Geometry check sheet. Reference: the model listing, model coordinates, mm. A direction names the side the tool comes from. Round coordinates to 2 decimals unless told otherwise and drop trailing zeros. Loops run counter-clockwise (first coordinate to the right, second up) from the corner with the lowest first, then second, coordinate; pieces in that order, holes last. Notation, with made-up numbers: M 54.5,34 L 73.5,34 A19 ccw 73.5,65 Z; hole C -1,-21 d11. An arc over 180 degrees is marked long. Answer in a Markdown table with one row per item. Add a question column.
```python
from build123d import *

# Parameters (mm, degrees)
SKETCH1_R                = 9
SKETCH1_R_2              = 7
BOSS_EXTRUDE1_DEPTH      = 25
CUT_EXTRUDE2_DEPTH       = 12
CUT_EXTRUDE2_DEPTH_BACK  = 27
SKETCH2_R                = 9
BOSS_EXTRUDE8_DEPTH      = 9
BOSS_EXTRUDE8_DEPTH_BACK = 9
SKETCH4_R                = 9
SKETCH5_R                = 8
CUT_EXTRUDE3_DEPTH       = 3
CUT_EXTRUDE4_START       = -3
SKETCH6_R                = 8
CUT_EXTRUDE4_DEPTH       = 3
SKETCH7_R                = 2.5
CUT_EXTRUDE5_DEPTH       = 17
CUT_EXTRUDE6_DEPTH       = 15
FILLET2_R                = 1


with BuildPart() as part:
    # Sketch1 → Boss-Extrude1 (new body)
    with BuildSketch(Plane(origin=(0, 0, 0), x_dir=(1, 0, 0), z_dir=(0, 1, 0))):
        with Locations(Location((0, 0, 0), (0, 0, 270))):
            Circle(SKETCH1_R)
        with Locations(Location((0, 0, 0), (0, 0, 270))):
            Circle(SKETCH1_R_2, mode=Mode.SUBTRACT)
    extrude(amount=BOSS_EXTRUDE1_DEPTH)

    # Sketch2 → Cut-Extrude2 (cut, two sides: drawn at the far end of the back side and taken through both)
    with BuildSketch(Plane.XY.offset(9).offset(-CUT_EXTRUDE2_DEPTH_BACK)):
        with Locations((0, 25)):
            Circle(SKETCH2_R)
    extrude(amount=CUT_EXTRUDE2_DEPTH + CUT_EXTRUDE2_DEPTH_BACK, mode=Mode.SUBTRACT)

    # Sketch4 → Boss-Extrude8 (add, two sides: drawn at the far end of the back side and taken through both)
    with BuildSketch(Plane.XY.offset(-BOSS_EXTRUDE8_DEPTH_BACK)):
        with Locations((0, 25)):
            Circle(SKETCH4_R)
    extrude(amount=BOSS_EXTRUDE8_DEPTH + BOSS_EXTRUDE8_DEPTH_BACK)

    # Sketch5 → Cut-Extrude3 (cut)
    with BuildSketch(Plane.XY.offset(9)):
        with Locations((0, 25)):
            Circle(SKETCH5_R)
    extrude(amount=-CUT_EXTRUDE3_DEPTH, mode=Mode.SUBTRACT)

    # Sketch6 → Cut-Extrude4 (cut)
    with BuildSketch(Plane(origin=(0, 0, -9), x_dir=(-1, 0, 0), z_dir=(0, 0, -1)).offset(CUT_EXTRUDE4_START)):
        with Locations((0, 25)):
            Circle(SKETCH6_R)
    extrude(amount=CUT_EXTRUDE4_DEPTH, mode=Mode.SUBTRACT)

    # Sketch7 → Cut-Extrude5 (cut)
    with BuildSketch(Plane(origin=(0, 0, -6), x_dir=(-1, 0, 0), z_dir=(0, 0, -1))):
        with Locations((0, 25)):
            Circle(SKETCH7_R)
    extrude(amount=-CUT_EXTRUDE5_DEPTH, mode=Mode.SUBTRACT)

    # Sketch8 → Cut-Extrude6 (cut)
    with BuildSketch(Plane.XY.offset(6)):
        with BuildLine():
            Line((-10.5, 25), (-10.5, 14.5))
            Line((-10.5, 14.5), (10.5, 14.5))
            Line((10.5, 14.5), (10.5, 25))
            ThreePointArc((10.5, 25), (0, 35.5), (-10.5, 25))
        make_face()
    cut_extrude6 = extrude(amount=CUT_EXTRUDE6_DEPTH, mode=Mode.SUBTRACT)

    # Mirror1: Cut-Extrude6 across plane
    add(cut_extrude6.mirror(Plane.XY), mode=Mode.SUBTRACT)

    # Fillet2
    fillet2_edges = [part.edges().sort_by_distance(p)[0] for p in [
        (0, 14.5, -9),
        (-6.708203932, 16.75, -6),
        (6.708203932, 16.75, -6),
        (6.708203932, 16.75, 6),
        (-6.708203932, 16.75, 6),
        (-3.674234614, 14.5, 8.215838363),
    ]]
    fillet(fillet2_edges, radius=FILLET2_R)


solid = part.part
```
1) Cross-section at C-C, the plane y = 11. Record the boundary of the cut face in (x, z), plus the area to 3 significant figures.
2) Set-up check for faces 1 (the cylindrical face through (2.703, 9.547, 8.584)), 2 (the flat face through (-7.3, 0, 0)): record each of +Z, -Z, +X, -X, +Y, -Y from which the full face is reachable in a straight line by a thin tool's end or side.
3) Cross-section at D-D, the plane x = 7.5. Record the boundary of the cut face in (y, z).
4) Cross-section at A-A, the plane x = 0. Record the boundary of the cut face in (y, z).
5) Thickness scan on L1, parallel to X at y = 9, z = 0; L2, parallel to Z at x = -4.75, y = 26; L3, parallel to Y at x = 0.5, z = -5. Record the ranges inside material, lowest first. Write a range as [from, to].
6) Draft check along Y on faces 3 (the cylindrical face through (0.33, 27.48, -0.08)), 4 (the flat face through (-0.1, 14.5, 7.2)), 5 (the cylindrical face through (0, 10, -7)), 6 (the cylindrical face through (0, 34, 0)). Enter one of: +Y half, -Y half, draft (parallel to the pull), parting line (faces both ways), or undercut.
7) Go/stop test with flat-tipped pins: pin 1 (4 mm diameter, centred on x = -2, y = 17, fed in from -Z); pin 2 (4 mm diameter, centred on x = 4.5, z = 0.5, fed in from -Y); pin 3 (3 mm diameter, centred on y = 23, z = 2.5, fed in from +X). Record where each tip stops, or that it passes through.
8) Cross-section at B-B, the plane z = 4.25. Record the boundary of the cut face in (x, y).
Worked answers:
| question | item | result |
|---|---|---|
| 1 | outline | C 0,0 d18; hole C 0,0 d14 |
| 1 | area | 101 mm2 |
| 2 | face 1 | -Y |
| 2 | face 2 | +Z, -Z, +X, -X, -Y |
| 3 | outline | M 0,-4.97 L 20.03,-4.97 L 20.03,-6 L 29.97,-6 L 29.97,6 L 20.03,6 L 20.03,4.97 L 0,4.97 Z |
| 4 | outline | M 0,-9 L 13.5,-9 A1 ccw 14.5,-8 L 14.5,-7 L 0,-7 Z; M 0,7 L 14.5,7 L 14.5,8 A1 ccw 13.5,9 L 0,9 Z; M 16,-6 L 22.5,-6 L 22.5,6 L 16,6 Z; M 27.5,-6 L 34,-6 L 34,6 L 27.5,6 Z |
| 5 | L1 | x = [-9, -7], [7, 9] |
| 5 | L2 | z = [-6, 6] |
| 5 | L3 | y = [16.01, 22.55], [27.45, 33.99] |
| 6 | face 3 | undercut |
| 6 | face 4 | +Y half |
| 6 | face 5 | draft |
| 6 | face 6 | parting line |
| 7 | pin 1 | stops at z = -6 |
| 7 | pin 2 | stops at y = 16.35 |
| 7 | pin 3 | stops at x = 8.99 |
| 8 | outline | M -7.93,0 L -5.56,0 L -5.56,17.92 A9 ccw 5.56,17.92 L 5.56,0 L 7.93,0 L 7.93,20.75 A9 ccw long -7.93,20.75 Z; hole C 0,25 d5 |
